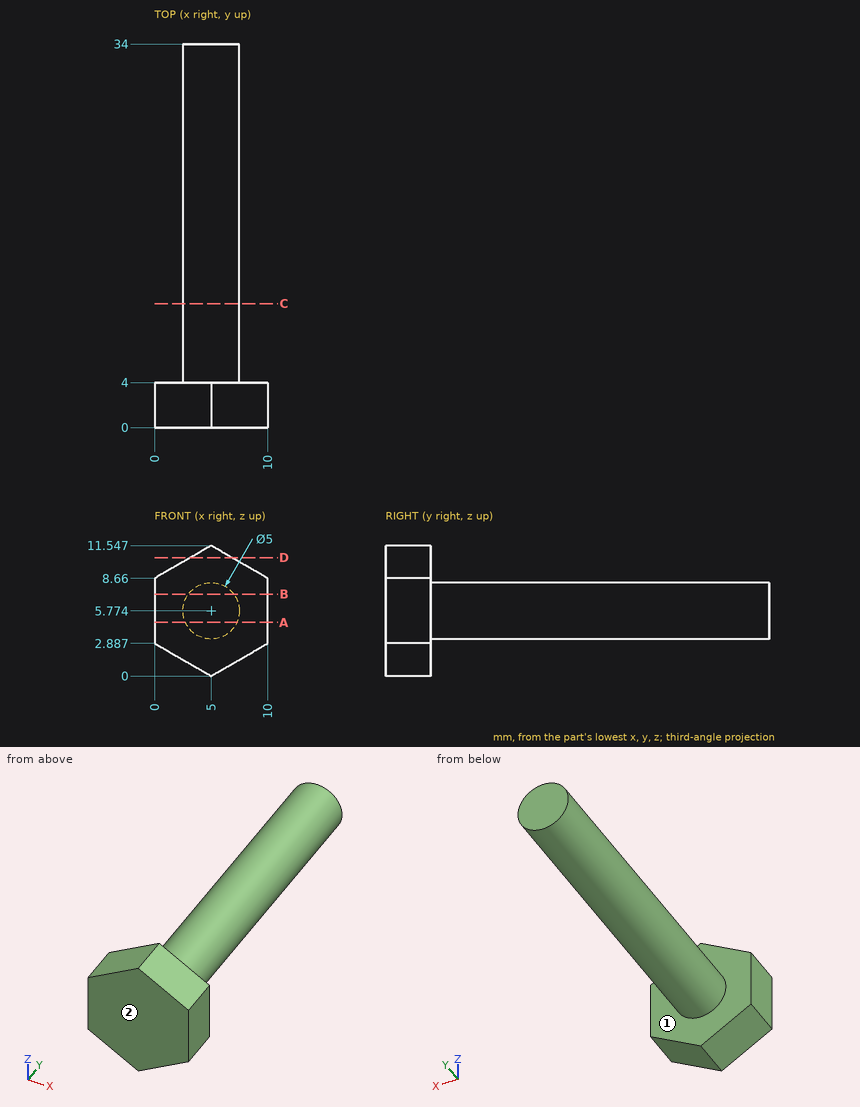
Input: dimensioned drawing with shaded views. Units: mm. Origin: part minimum x, y, z. A direction names the side the tool comes from. Coordinates: 2 decimals unless noted, no trailing zeros. Order: outer loops, then holes, each group sorted by start corner. A loop starts at its lowest first (then second) coordinate and runs counter-clockwise, first axis right, second up. Notation, with made-up numbers: (74.25, 8.5) - (83.25, 8.5) arc R29 ccw to (83.25, 43.5) - close; hole circle Ø3 at (59.5, 54.5). An arc over 180 degrees is marked (long way). Put each result on its own line as item: value.
1. Line query: line 1 along Z through (x, y) = (5, 20.5); line 2 along Y through (x, z) = (4.5, 8.5); line 3 along Z through (x, y) = (9.75, 3.5) (1 decimal). Output: solid intervals per line, ascending.
Report:
line 1: z = 3.27 to 8.27
line 2: y = 0 to 4
line 3: z = 2.7 to 8.8
2. Cut plane C-C on y = 11. Return the cut outline in (x, z).
Report:
outline: circle Ø5 at (5, 5.77)
3. Cut plane D-D on z = 10.5. Return the cut outline in (x, y), then the cut area to 3 significant figures.
Report:
outline: (3.19, 0) - (6.81, 0) - (6.81, 4) - (3.19, 4) - close
area: 14.5 mm2
4. Cut plane B-B on z = 7.25. Return the cut outline in (x, y), then the cut area to 3 significant figures.
Report:
outline: (0, 0) - (10, 0) - (10, 4) - (7.02, 4) - (7.02, 34) - (2.98, 34) - (2.98, 4) - (0, 4) - close
area: 161 mm2
5. Contact query for flat-ended pins moving along their axis: pin 1 Ø3 at (x, y) = (3, 27) entering from -Z; pin 2 Ø5 at (x, y) = (8.5, 17.5) entering from +Z (1 decimal); pin 3 Ø5 at (x, y) = (3.5, 13.5) entering from +Z. Output: stop coordinate, or through.
Report:
pin 1: stops at z = 3.32
pin 2: stops at z = 8.1
pin 3: stops at z = 8.27
6. Cut plane A-A on z = 4.75. Return the cut outline in (x, y).
Report:
outline: (0, 0) - (10, 0) - (10, 4) - (7.28, 4) - (7.28, 34) - (2.72, 34) - (2.72, 4) - (0, 4) - close
7. Reachability of the marked faces 1 and 2 from +Z, -Z, +X, -X, +Y, -Y: full face, straight path, thin tool, end or side. Return the list, or none.
Report:
face 1: +Y
face 2: +Z, -Z, +X, -X, -Y
